Design review of the part built by this model. Coordinates are the model's own, in mm. A direction names the side the tool comes from. Round coordinates to 2 decimals unless told otherwise and drop trailing zeros. Write each loop counter-clockwise with the first axis right and the second up, starting at its lowest first coordinate (ties: lowest second). Pieces come first, ordered by that corner, then holes. Notation, with made-up numbers: (-37, 56) - (13, 56) arc R19 ccw to (13, 61) - close; hole circle Ø7 at (37.5, 85). An arc over 180 degrees is marked (long way). Use one line per item in the form item = value.
```python
from build123d import *

# Parameters (mm, degrees)
SKETCH1_R           = 2.5
SKETCH1_R_2         = 1
BOSS_EXTRUDE1_DEPTH = 2
BOSS_EXTRUDE2_DEPTH = 0.8
CUT_EXTRUDE1_DEPTH  = 14.872182458


with BuildPart() as part:
    # Sketch1 → Boss-Extrude1 (new body)
    with BuildSketch(Plane(origin=(0, 0, 0), x_dir=(1, 0, 0), z_dir=(0, 1, 0))):
        with Locations(Location((0, 0, 0), (0, 0, 270))):
            Circle(SKETCH1_R)
        with Locations(Location((0, 0, 0), (0, 0, 270))):
            Circle(SKETCH1_R_2, mode=Mode.SUBTRACT)
    extrude(amount=BOSS_EXTRUDE1_DEPTH)

    # Sketch7 → Boss-Extrude2 (add, symmetric)
    with BuildSketch(Plane(origin=(-0.8, 0, 0), x_dir=(0, -1, 0), z_dir=(-1, 0, 0))):
        with BuildLine():
            Line((1.954019719, 6.809600844), (1.954019719, 12.409600844))
            ThreePointArc((1.954019719, 12.409600844), (1.321034736, 13.059378105), (0.654910522, 12.443619215))
            Line((0.654910522, 12.443619215), (0.361426958, 6.843619215))
            ThreePointArc((0.361426958, 6.843619215), (0.301852122, 6.612668496), (0.157008946, 6.423174828))
            ThreePointArc((0.157008946, 6.423174828), (-1.158621723, 4.654463774), (-1.625, 2.5))
            Line((-1.625, 2.5), (-1.625, 1.75))
            Line((-1.625, 1.75), (-0.375, 1.75))
            Line((-0.375, 1.75), (-0.375, 2.5))
            ThreePointArc((-0.375, 2.5), (-0.11625091, 3.523019396), (0.597766538, 4.3))
            ThreePointArc((0.597766538, 4.3), (1.593265867, 5.383283989), (1.954019719, 6.809600844))
        make_face()
    extrude(amount=BOSS_EXTRUDE2_DEPTH, both=True)

    # Sketch9 → Cut-Extrude1 (cut, through all)
    with BuildSketch(Plane.XZ.offset(1.954019719)):
        Polygon((0, 2.5), (-0.3, 7.71372429), (0, 7.71372429), align=None)
    extrude(amount=-CUT_EXTRUDE1_DEPTH, mode=Mode.SUBTRACT)


solid = part.part
```
Q1. To check wall thickness, follow line 1 along X through (y, z) = (0.8, 0); line 2 along Y through (x, z) = (1.65, 1); line 3 along Z through (x, y) = (0.8, 0.85). State the ranges of each line that lie inside material, in increasing order. Write a range as from..to.
Calculated:
line_1 = -2.5..-1, 1..2.5
line_2 = 0..2
line_3 = -2.37..-0.6, 0.6..2.37
Q2. Machinability: for faces 5 (the flat face through (-0.148, -0.19, 5.07)), 6 (the cylindrical face through (-0.811, 0.123, 3.51)), 7 (the flat face through (-1, 0, 1)), 8 (the flat face through (-1, 2, 1)), which of the approach directions +Z, -Z, +X, -X, +Y, -Y give a long, thin tool a straight path to every point of the face, cutting with its end or side? Answer none if there is none.
Calculated:
face_5 = +X, +Y, -Y
face_6 = +X, -X, -Y
face_7 = -Z, +X, -X, -Y
face_8 = +Z, -Z, +X, -X, +Y
Q3. Draft analysis for pull direction X (two halves, no side actions). For faces 1 (the cylindrical face through (0.1, 1, -2.5)), 2 (the flat face through (-1.6, -1, 8)), 3 (the flat face through (-0.81, -0.51, 9.68)), 4 (the cylindrical face through (-1, 1, 0)), state which applies: released by +X, released by -X, zero draft, split by the parting line, or undercut.
Calculated:
face_1 = split by the parting line
face_2 = released by -X
face_3 = zero draft
face_4 = undercut
Q4. We need section A-A on z = 0. Write out the cut boundary in (x, y).
Calculated:
outline = (-2.5, 0) - (-1, 0) - (-1, 2) - (-2.5, 2) - close; (1, 0) - (2.5, 0) - (2.5, 2) - (1, 2) - close
Q5. We need section D-D on z = 1.75. Write out the cut boundary in (x, y).
Calculated:
outline = (-1.79, 0) - (1.79, 0) - (1.79, 2) - (-1.79, 2) - close
Q6. We need section B-B on x = 0.35. Write out the cut boundary in (y, z).
Calculated:
outline = (0, -2.48) - (2, -2.48) - (2, -0.94) - (0, -0.94) - close; (0, 0.94) - (2, 0.94) - (2, 2.48) - (0, 2.48) - close
Q7. For P1, Ø2, axis at x = -1, y = 1, coming from the -Z side; P2, Ø1, axis at y = 1.5, z = 7, coming from the -X side; P3, Ø2.5, axis at x = 0.5, z = 1, coming from the -Y side; P4, Ø1.2, axis at y = -1, z = 10, coming from the +X side, all flat-tipped, find the tip position at first contact; note any pin that passes through.
Calculated:
P1 = -2.5
P2 = through
P3 = 0
P4 = 0
Q8. We need section C-C on y = -1.1. Write out the cut boundary in (x, z), then the cut area to 3 significant figures.
Calculated:
outline = (-1.6, 4.71) - (-0.13, 4.71) - (-0.3, 7.71) - (0, 7.71) - (0, 13.03) - (-1.6, 13.03) - close
area = 12.7 mm2
